```python
from build123d import *

# Parameters (mm, degrees)
SCALE1_SCALE = 649.76746201
SHELL2_T     = 5.588


with BuildPart() as part:
    # Sketch1 → Revolve2 (revolve)
    with BuildSketch(Plane.XY):
        with BuildLine():
            Line((0.30325, 0.129), (-0.275595218, 0.129))
            ThreePointArc((-0.275595218, 0.129), (-0.3184401, 0.116916493), (-0.348657753, 0.084227221))
            Line((-0.348657753, 0.084227221), (-0.372858421, 0.036730735))
            ThreePointArc((-0.372858421, 0.036730735), (-0.374701425, 0.034736985), (-0.377314576, 0.034))
            Line((-0.377314576, 0.034), (-0.40125, 0.034))
            Line((-0.40125, 0.034), (-0.40125, 0))
            Line((-0.40125, 0), (0.40125, 0))
            Line((0.40125, 0), (0.40125, 0.000587576))
            ThreePointArc((0.40125, 0.000587576), (0.399958659, 0.015347671), (0.396123873, 0.029659288))
            Line((0.396123873, 0.029659288), (0.379365102, 0.075703632))
            ThreePointArc((0.379365102, 0.075703632), (0.349709691, 0.114351316), (0.30325, 0.129))
        make_face()
    revolve(axis=Axis((-0.40125, 0, 0), (1, 0, 0)))


with BuildPart() as part_1:
    # Scale1: scaled about (0, 0, 0)
    add(part.part.scale(SCALE1_SCALE))

    # Shell2 (no face opened: a closed hollow body)
    add(offset(amount=-SHELL2_T, mode=Mode.PRIVATE), mode=Mode.SUBTRACT)


solid = part_1.part
```
Geometry: final body of the model. Coordinates: model frame, mm. A direction names the side the tool comes from. Coordinates: 2 decimals unless noted, no trailing zeros. Order: outer loops, then holes, each group sorted by start corner. A loop starts at its lowest first (then second) coordinate and runs counter-clockwise, first axis right, second up. Notation, with made-up numbers: (-15.5, 54) -> (-7.5, 54) arc R18 cw to (-7.5, 76) -> close; hole circle Ø3 at (-28, 5). An arc over 180 degrees is marked (long way). Use CSV: the item, a comma, the result in double quotes.
1) Pin query (flat end, axial travel): pin 1 Ø1 at (y, z) = (-7, 40.5) entering from +X; pin 2 Ø1 at (x, y) = (101.5, -19.5) entering from -Z; pin 3 Ø5 at (y, z) = (13.5, -15) entering from +X. Return the tip coordinate at first contact, or that it passes through.
Findings:
pin 1,"stops at x = 249.63"
pin 2,"stops at z = -81.64"
pin 3,"stops at x = 257.94"
2) Access query for faces 4 (the flat face through (-260.719, 0, 0)), 5 (the cylindrical face through (-253.052, -4.789, -21.567)), 6 (the cylindrical face through (-250.22, 15.74, 4.96)). Directions: +Z, -Z, +X, -X, +Y, -Y. A direction counts if a zero-diameter tool reaches every point of the face in a straight line with its end or side. Return the directions, or none.
Findings:
face 4,"+Z, -Z, -X, +Y, -Y"
face 5,"-X"
face 6,"none"
3) Section A-A on x = 123. Output: boundary loops of the cut face in (y, z), then the cut area to 3 significant figures.
Findings:
outline,"circle Ø167.64 at (0, 0); hole circle Ø156.46 at (0, 0)"
area,"2,840 mm^2"
4) Line query: line 1 (Z direction, x = -101, y = 0); line 2 (Z direction, x = -251.5, y = 0); line 3 (X direction, y = 2, z = 0). Output: solid intervals per line, ascending.
Findings:
line 1,"z = -83.82 to -78.23, 78.23 to 83.82"
line 2,"z = -22.09 to -16.5, 16.5 to 22.09"
line 3,"x = -260.72 to -255.13, 255.1 to 260.7"
5) Mould query, pull axis X, two halves, no side actions, for faces 1 (the cylindrical face through (6.35, -16.96, -76.37)), 2 (the cylindrical face through (6.352, -18.171, -81.827)), 3 (the conical face through (256.707, -4.583, -20.64)). Classes: +X half, -X half, draft (parallel to the pull), parting line (faces both ways), or undercut.
Findings:
face 1,"undercut"
face 2,"draft"
face 3,"+X half"
